Answer from the drawing. Dimensions are ordinates in mm from the lowest x, y and z of the part. A direction names the side the tool comes from. Give positions to 0.01 mm unless a question says otherwise; leave off trailing zeros. Write each loop counter-clockwise with the first axis right and the second up, starting at its lowest first coordinate (ties: lowest second). Pieces come first, ordered by that corner, then holes.
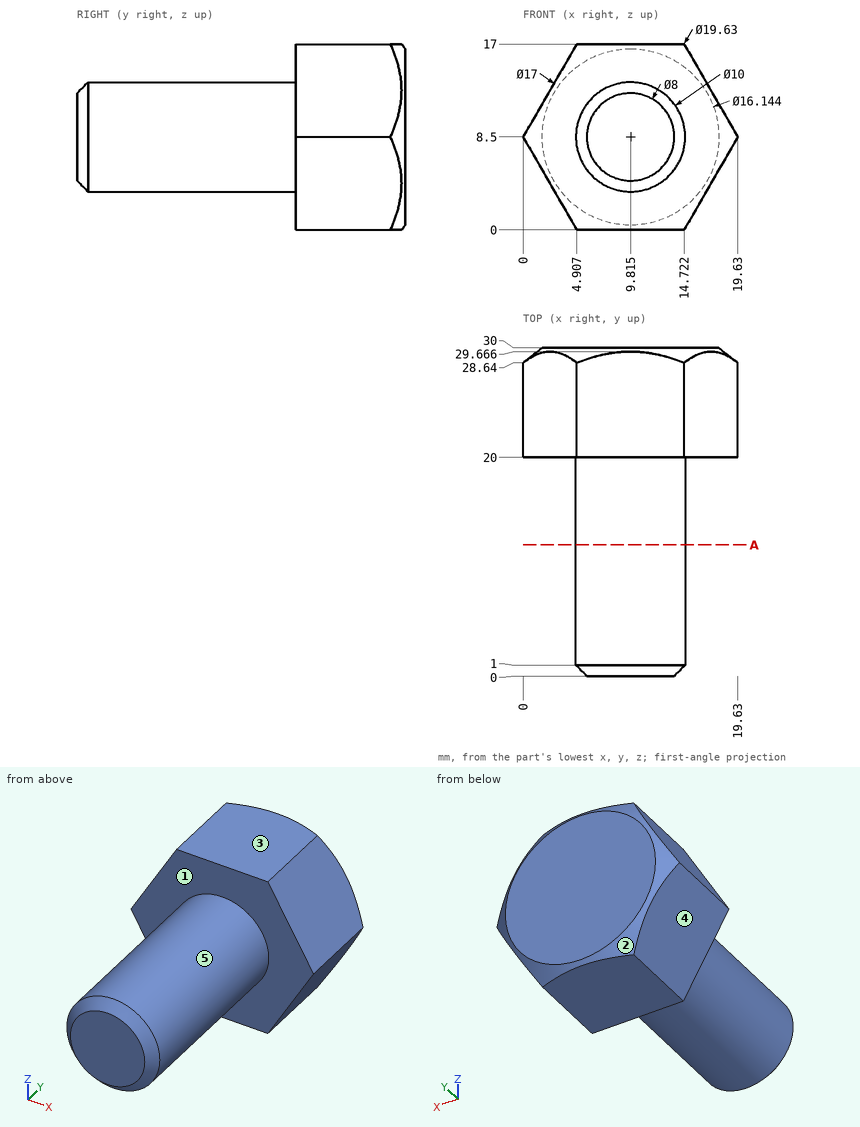
Item 1: Determine the mould class of the marked faces 3, 4 and 5 for opening direction X: pulls with the +X half, pulls with the -X half, needs draft (parallel to the pull), parting line crosses it, or undercut.
Result set:
face 3: needs draft
face 4: pulls with the -X half
face 5: parting line crosses it
Item 2: Each of these flat-tipped pins is pushed along its axis until it touches: pin 1 Ø4 at (x, y) = (2.5, 21) entering from +Z (1 decimal); pin 2 Ø5 at (y, z) = (7, 13) entering from -X; pin 3 Ø10 at (x, y) = (13, 13) entering from -Z. Where does it stop, or does it pass through?
Result set:
pin 1: stops at z = 16.3
pin 2: stops at x = 5.23
pin 3: stops at z = 3.5
Item 3: Section A-A (y = 12) is taken. Write down the section's boundary in (x, z) (1 decimal).
Result set:
outline: circle Ø10 at (9.8, 8.5)
Item 4: Find the intervals of material crossed by line 1 along X through (y, z) = (3.5, 8.25); line 2 along Y through (x, z) = (9.75, 14); line 3 along Z through (x, y) = (11, 19.25), in increasing order.
Result set:
line 1: x = 4.82 to 14.81
line 2: y = 20 to 30
line 3: z = 3.64 to 13.36
Item 5: Which of the six approach directions +Z, -Z, +X, -X, +Y, -Y give full straight-line access (tool end or side, diameter ignored) to the marked faces 1 and 2?
Result set:
face 1: -Y
face 2: +Y
